from build123d import *

# Parameters (mm, degrees)
F0_W      = 24.1681
F0_H      = 25.4
F1_DEPTH  = 5.08
F2_R      = 9.84758
F3_DEPTH  = 2.54
F4_R      = 10.706062
F4_R_2    = 9.84758
F5_DEPTH  = 0.6858
F6_W      = 5.08
F6_H      = 2.54
F7_DEPTH  = 6.35
F8_W      = 2.54
F8_H      = 2.54
F9_DEPTH  = 0.254
F10_R     = 0.508
F11_W     = 2.54
F11_H     = 2.54
F12_DEPTH = 0.254
F13_R     = 0.508


with BuildPart() as f1:
    # F0 (on Top) → F1 (new body)
    with BuildSketch(Plane.XY):
        Rectangle(F0_W, F0_H)
    extrude(amount=F1_DEPTH)

    # F2 (on Top) → F3 (cut)
    with BuildSketch(Plane.XY):
        Circle(F2_R)
    extrude(amount=F3_DEPTH, mode=Mode.SUBTRACT)

    # F4 (on face) → F5 (cut)
    with BuildSketch(Plane(origin=(0, 0, 2.54), x_dir=(1, 0, 0), z_dir=(0, 0, -1))):
        Circle(F4_R)
        Circle(F4_R_2, mode=Mode.SUBTRACT)
    extrude(amount=F5_DEPTH, mode=Mode.SUBTRACT)

    # F6 (on face) → F7 (join)
    with BuildSketch(Plane.YZ.offset(12.08405)):
        with Locations((0, 1.27)):
            Rectangle(F6_W, F6_H)
    extrude(amount=F7_DEPTH)

    # F8 (on face) → F9 (join)
    with BuildSketch(Plane.XZ.offset(2.54)):
        with Locations((17.16405, 1.27)):
            Rectangle(F8_W, F8_H)
    extrude(amount=F9_DEPTH)

    # F10
    f10_edges = [f1.edges().sort_by_distance(p)[0] for p in [
        (18.43405, -2.794, 1.27),
    ]]
    fillet(f10_edges, radius=F10_R)

    # F11 (on face) → F12 (join)
    with BuildSketch(Plane(origin=(0, 2.54, 0), x_dir=(-1, 0, 0), z_dir=(0, 1, 0))):
        with Locations((-17.16405, 1.27)):
            Rectangle(F11_W, F11_H)
    extrude(amount=F12_DEPTH)

    # F13
    f13_edges = [f1.edges().sort_by_distance(p)[0] for p in [
        (18.43405, 2.794, 1.27),
    ]]
    fillet(f13_edges, radius=F13_R)


solid = f1.part
Model file for the job. Use its own axes, mm. A direction names the side the tool comes from. Round coordinates to 2 decimals unless told otherwise and drop trailing zeros. Order: outer loops, then holes, each group sorted by start corner. A loop starts at its lowest first (then second) coordinate and runs counter-clockwise, first axis right, second up. Notation, with made-up numbers: M 54,9 L 98,9 A22 cw 98,19 Z; hole C -37,41.5 d9. An arc over 180 degrees is marked long. Write each question's results on one line, items separated by ' | '. Start each with the question number.
(1) Which spindle directions (+Z, -Z, +X, -X, +Y, -Y) get a long thin tool onto all of the face, cutting with end or side? Do faces 4 (the face through (17, -2.794, 1)), 5 (the face through (4.54, -8.74, 0.91)), 6 (the face through (14, 2.54, 1)). Say none if no direction does.
(2) Saw through at B-B, the plane x = 0. Give the cut face in (y, z).
(3) Saw through at D-D, the plane z = 2.9. Give the cut face in (x, y).
(4) Probe probe 1 along X at (y, z) = (0, 2); probe 2 along Y at (x, z) = (0, 2.2); probe 3 along X at (y, z) = (0, 0.65). List the from-to ranges inside material, lowest first. Write a range as from..to.
(5) Saw through at C-C, the plane y = 0. Give the cut face in (x, z), then the cut area to 3 significant figures.
(6) Saw through at A-A, the plane z = 1.4. Give the cut face in (x, y).
(7) Two-plate mould, pull along Y, no slides. Class faces 1 (the face through (15, 0, 2.54)), 2 (the face through (14, -2.54, 1)), 3 (the face through (5, 9, 1.854)): pulls with the +Y half, pulls with the -Y half, needs draft (parallel to the pull), parting line crosses it, or undercut.
(8) Drop flat-ended pins along their axis: pin 1 (12 mm diameter, centred on x = 12.5, y = -9, fed in from +Z); pin 2 (0.6 mm diameter, centred on x = 17.5, z = 1, fed in from -Y); pin 3 (0.8 mm diameter, centred on x = 13, z = 1.5, fed in from -Y); pin 4 (1.6 mm diameter, centred on x = 17, z = 1.5, fed in from +Y). Give the stop position or say it passes through.
Established:
1) face 4: +Z, -Z, +X, -Y | face 5: -Z | face 6: +Z, -Z, +Y
2) outline: M -12.7,0 L -9.85,0 L -9.85,1.85 L -10.71,1.85 L -10.71,2.54 L 10.71,2.54 L 10.71,1.85 L 9.85,1.85 L 9.85,0 L 12.7,0 L 12.7,5.08 L -12.7,5.08 Z
3) outline: M -12.08,-12.7 L 12.08,-12.7 L 12.08,12.7 L -12.08,12.7 Z
4) probe 1: x = -12.08..-10.71, 10.71..18.43 | probe 2: y = -12.7..-10.71, 10.71..12.7 | probe 3: x = -12.08..-9.85, 9.85..18.43
5) outline: M -12.08,0 L -9.85,0 L -9.85,1.85 L -10.71,1.85 L -10.71,2.54 L 10.71,2.54 L 10.71,1.85 L 9.85,1.85 L 9.85,0 L 18.43,0 L 18.43,2.54 L 12.08,2.54 L 12.08,5.08 L -12.08,5.08 Z | area: 87.7 mm^2
6) outline: M -12.08,-12.7 L 12.08,-12.7 L 12.08,-2.54 L 15.89,-2.54 L 15.89,-2.79 L 17.93,-2.79 A0.51 ccw 18.43,-2.29 L 18.43,2.29 A0.51 ccw 17.93,2.79 L 15.89,2.79 L 15.89,2.54 L 12.08,2.54 L 12.08,12.7 L -12.08,12.7 Z; hole C 0,0 d19.7
7) face 1: needs draft | face 2: pulls with the -Y half | face 3: undercut
8) pin 1: stops at z = 5.08 | pin 2: stops at y = -2.79 | pin 3: stops at y = -2.54 | pin 4: stops at y = 2.79
